```python
from build123d import *

# Parameters (mm, degrees)
SKETCH2_R          = 6
CUT_EXTRUDE1_DEPTH = 23.315913604
FILLET1_R          = 0.25


with BuildPart() as part:
    # Sketch1 → Revolve2 (revolve)
    with BuildSketch(Plane(origin=(0, 0, 0), x_dir=(0, 0, -1), z_dir=(1, 0, 0))):
        with BuildLine():
            Line((0, -8), (7.549834435, -8))
            ThreePointArc((7.549834435, -8), (11, 0), (7.549834435, 8))
            Line((7.549834435, 8), (0, 8))
            Line((0, 8), (0, -8))
        make_face()
    revolve(axis=Axis((0, 11, 0), (0, -1, 0)))

    # Sketch2 → Cut-Extrude1 (cut, through all)
    with BuildSketch(Plane(origin=(0, 8, 0), x_dir=(1, 0, 0), z_dir=(0, 1, 0))):
        with Locations(Location((0, 0, 0), (0, 0, 270))):
            Circle(SKETCH2_R)
    extrude(amount=-CUT_EXTRUDE1_DEPTH, mode=Mode.SUBTRACT)

    # Fillet1
    fillet1_edges = [part.edges().sort_by_distance(p)[0] for p in [
        (0, -8, -6),
        (0, 8, -6),
        (0, -8, 7.549834435),
        (0, 8, 7.549834435),
    ]]
    fillet(fillet1_edges, radius=FILLET1_R)


solid = part.part
```
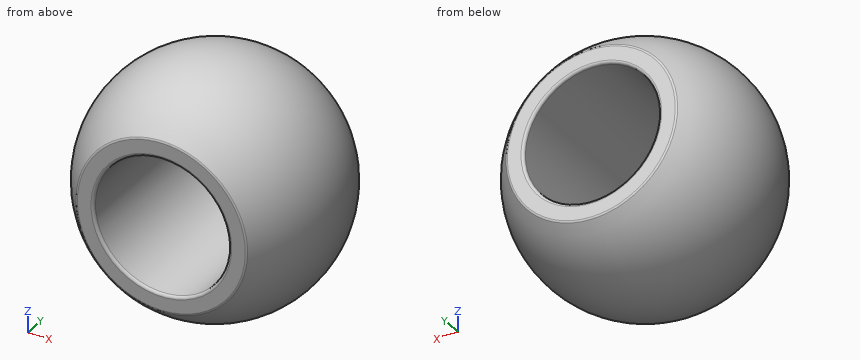
Check sheet for the modelled part. Datum: model origin and axes. Units: mm. Give positions to 0.01 mm unless a question says otherwise; leave off trailing zeros. Write each loop counter-clockwise with the first axis right and the second up, starting at its lowest first coordinate (ties: lowest second). Pieces come first, ordered by that corner, then holes.
Item 1: Scan lines: L1, parallel to Z at x = 5.25, y = 0; L2, parallel to Z at x = 2.5, y = -2; L3, parallel to X at y = 6, z = -0.75. Record each from-to range of solid material in increasing order.
Item 2: Cross-section at D-D (z = -9.5). Enter the section's corners in (x, y), and give its area (3 significant figures).
Item 3: Cross-section at A-A (y = 5.25). Enter the section's corners in (x, z), and give its area (3 significant figures).
Item 4: Cross-section at B-B (z = 8.75). Enter the section's corners in (x, y).
Item 5: Cross-section at C-C (y = 2.5). Enter the section's corners in (x, z).
Item 6: Gauge pin test, flat ends, axial feed: pin 1 (3 mm diameter, centred on x = -5.5, y = -2.5, fed in from -Z); pin 2 (8 mm diameter, centred on y = -3.5, z = -7.5, fed in from +X); pin 3 (4 mm diameter, centred on x = 7.5, y = -2.5, fed in from +Z); pin 4 (9.5 mm diameter, centred on x = 0, z = 0, fed in from +Y). Record the tip position at first contact, or that the pin passes through.
Report:
1. L1: z = -9.67 to -2.9, 2.9 to 9.67
1. L2: z = -10.52 to -5.45, 5.45 to 10.52
1. L3: x = -9.19 to -5.95, 5.95 to 9.19
2. outline: circle Ø11.09 at (0, 0)
2. area: 96.6 mm2
3. outline: circle Ø19.33 at (0, 0); hole circle Ø12 at (0, 0)
3. area: 180 mm2
4. outline: circle Ø13.33 at (0, 0)
5. outline: circle Ø21.42 at (0, 0); hole circle Ø12 at (0, 0)
6. pin 1: stops at z = -10.02
6. pin 2: stops at x = 10.13
6. pin 3: stops at z = 9.28
6. pin 4: passes through
